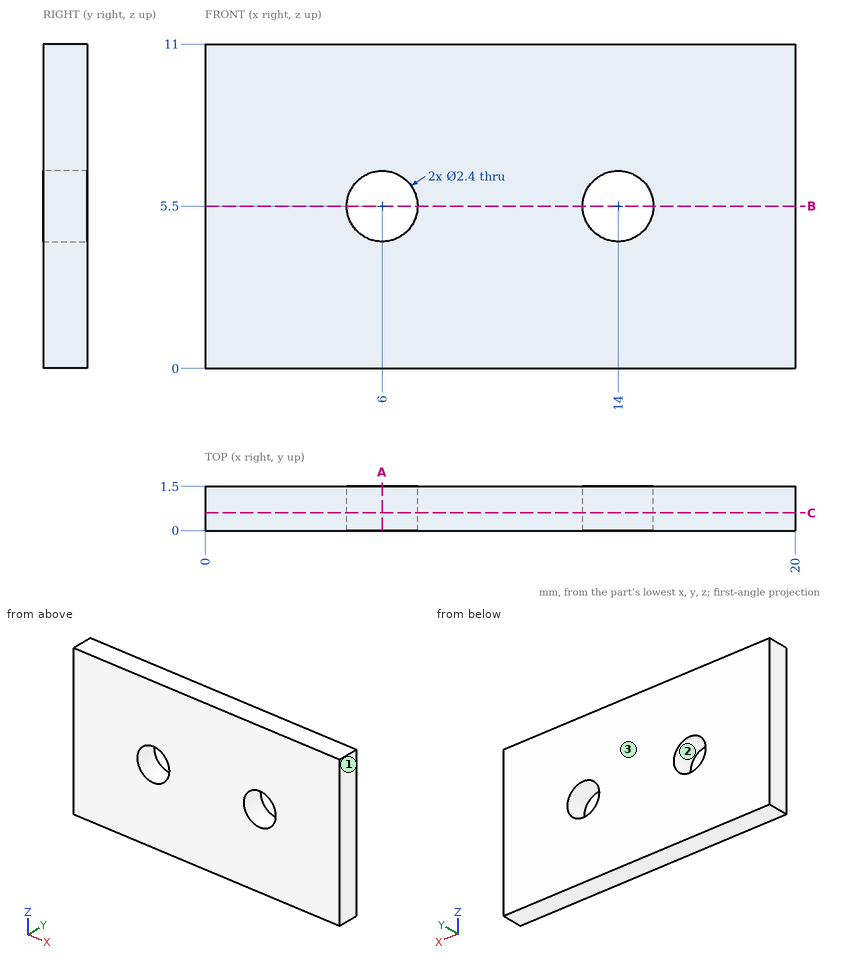
Can you work these out from the drawing? Everything is in mm from the part's minimum corner. Coordinates: 2 decimals unless noted, no trailing zeros. Write each loop counter-clockwise with the first axis right and the second up, starting at its lowest first coordinate (ties: lowest second). Pieces come first, ordered by that corner, then holes. Notation, with made-up numbers: (1, 20) -> (9, 20) arc R18 cw to (9, 49) -> close; hole circle Ø3 at (53.25, -38.5). An arc over 180 degrees is marked (long way). Write each question's results on one line, items separated by ' | '. Start each with the question number.
Item 1: Please list where these lines run through material, in increasing order: probe 1 along X at (y, z) = (0.55, 5.5); probe 2 along Z at (x, y) = (6.5, 1.4); probe 3 along Z at (x, y) = (13.25, 1).
Item 2: Thinking about a two-plate mould opening in X: for the marked faces 1, 2 and 3, which applies, released by +X, released by -X, zero draft, split by the parting line, or undercut?
Item 3: If we section it at C-C, the plane y = 0.6: Write out the boundary of the cut face in (x, z), and give its area (3 significant figures).
Item 4: If we section it at B-B, the plane z = 5.5: Write out the boundary of the cut face in (x, y), and give its area (3 significant figures).
Item 5: If we section it at A-A, the plane x = 6: Write out the boundary of the cut face in (y, z).
Answer block:
1) probe 1: 0 to 4.8, 7.2 to 12.8, 15.2 to 20 | probe 2: 0 to 4.41, 6.59 to 11 | probe 3: 0 to 4.56, 6.44 to 11
2) face 1: released by +X | face 2: undercut | face 3: zero draft
3) outline: (0, 0) -> (20, 0) -> (20, 11) -> (0, 11) -> close; hole circle Ø2.4 at (6, 5.5); hole circle Ø2.4 at (14, 5.5) | area: 211 mm²
4) outline: (0, 0) -> (4.8, 0) -> (4.8, 1.5) -> (0, 1.5) -> close; (7.2, 0) -> (12.8, 0) -> (12.8, 1.5) -> (7.2, 1.5) -> close; (15.2, 0) -> (20, 0) -> (20, 1.5) -> (15.2, 1.5) -> close | area: 22.8 mm²
5) outline: (0, 0) -> (1.5, 0) -> (1.5, 4.3) -> (0, 4.3) -> close; (0, 6.7) -> (1.5, 6.7) -> (1.5, 11) -> (0, 11) -> close
